The listing builds one solid part. Answer for the finished solid, in the listing's coordinates (mm). Face numbers are marked on the shaded views. A direction names the side the tool comes from. Coordinates: 2 decimals unless noted, no trailing zeros. Order: outer loops, then holes, each group sorted by start corner. A loop starts at its lowest first (then second) coordinate and runs counter-clockwise, first axis right, second up. Notation, with made-up numbers: (62.25, -5.5) -> (97.25, -5.5) arc R6 ccw to (97.25, -1.5) -> close; hole circle Ø4 at (78.5, 6.5). An arc over 180 degrees is marked (long way). Write each question's results on one line, items separated by ' | '. Start each with the question number.
(1) The part is cut by section B-B, the plane x = -15. Give the vertices of the cut face in (y, z).
(2) The part is cut by section D-D, the plane y = 30. Give the vertices of the cut face in (x, z), then the cut area to 3 significant figures.
(3) A tool of negligible diameter and unlimited length cuts with its end or side. For the marked faces 4, 5, 6 and 7, from which of +Z, -Z, +X, -X, +Y, -Y can it reach the whole face along a straight path? Write none if from no direction.
(4) Determine the mould class of the marked faces 1, 2 and 3 for opening direction Z: +Z half, -Z half, draft (parallel to the pull), parting line (faces both ways), or undercut.
(5) Straight lines are drawn through the part: L1, parallel to Z at x = -15, y = 7.5; L2, parallel to Y at x = -14, z = 3.5; L3, parallel to Z at x = -17.5, y = 24.5. For each, find the intervals that lie inside material, in ascending order.
(6) The part is cut by section A-A, the plane z = 0. Give the vertices of the cut face in (x, y).
(7) Given pin 1 (5 mm diameter, centred on x = -15, z = 0, fed in from -Y); pin 2 (8 mm diameter, centred on x = -21, z = -4, fed in from +Y); pin 3 (11 mm diameter, centred on y = 16.5, z = 1, fed in from +X); pin 4 (12 mm diameter, centred on x = -29.5, z = -11.5, fed in from -Y), each flat-ended and moving along its own axis, determine where each tip first touches the part or whether it passes through.
(8) The part is cut by section C-C, the plane z = -9.5. Give the vertices of the cut face in (x, y), then the cut area to 3 significant figures.
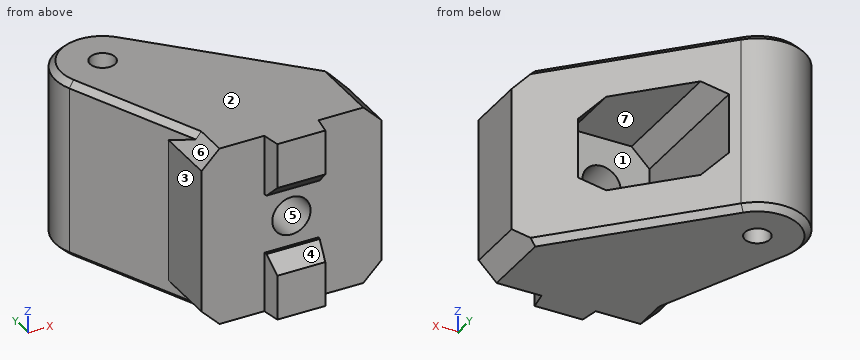
```python
from build123d import *

# Parameters (mm, degrees)
CROQUIS1_R              = 2.1
SALIENTE_EXTRUIR1_DEPTH = 15
CHAFL_N1_SIZE           = 3
CORTAR_EXTRUIR1_START   = -10
CROQUIS3_W              = 16
CROQUIS3_H              = 16
CORTAR_EXTRUIR1_DEPTH   = 28.9
CHAFL_N2_SIZE           = 3
CROQUIS4_R              = 3.2
CORTAR_EXTRUIR2_DEPTH   = 14
CROQUIS5_W              = 10
CROQUIS5_H              = 10
CORTAR_EXTRUIR3_DEPTH   = 4
CHAFL_N3_SIZE           = 2.5
CHAFL_N4_SIZE           = 1


with BuildPart() as part:
    # Croquis1 → Saliente-Extruir1 (new body, symmetric)
    with BuildSketch(Plane.XY):
        with BuildLine():
            Line((-30, 0), (-30, 10))
            Line((-30, 10), (-37.257580847, 26.8795))
            ThreePointArc((-37.257580847, 26.8795), (-34.35566426, 36.590765423), (-24.284119395, 35.453320907))
            Line((-24.284119395, 35.453320907), (0, 10))
            Line((0, 10), (0, 0))
            Line((0, 0), (-10.471019058, 0))
            Line((-10.471019058, 0), (-11, -3))
            Line((-11, -3), (-19, -3))
            Line((-19, -3), (-19.528980942, 0))
            Line((-19.528980942, 0), (-30, 0))
        make_face()
        with Locations((-30, 30)):
            Circle(CROQUIS1_R, mode=Mode.SUBTRACT)
    extrude(amount=SALIENTE_EXTRUIR1_DEPTH, both=True)

    # Chaflán1
    chafl_n1_edges = [part.edges().sort_by_distance(p)[0] for p in [
        (-30, 5, -15),
        (0, 5, -15),
        (-30, 5, 15),
        (0, 5, 15),
    ]]
    chamfer(chafl_n1_edges, length=CHAFL_N1_SIZE)

    # Croquis3 → Cortar-Extruir1 (cut, through all)
    with BuildSketch(Plane.XZ.offset(CORTAR_EXTRUIR1_START)):
        with Locations((-15, 0)):
            Rectangle(CROQUIS3_W, CROQUIS3_H)
    extrude(amount=-CORTAR_EXTRUIR1_DEPTH, mode=Mode.SUBTRACT)

    # Chaflán2
    chafl_n2_edges = [part.edges().sort_by_distance(p)[0] for p in [
        (-23, 22.053687666, -8),
        (-23, 22.053687666, 8),
        (-7, 13.668513637, 8),
        (-7, 13.668513637, -8),
    ]]
    chamfer(chafl_n2_edges, length=CHAFL_N2_SIZE)

    # Croquis4 → Cortar-Extruir2 (cut, through all)
    with BuildSketch(Plane(origin=(0, 10, 0), x_dir=(1, 0, 0), z_dir=(0, 1, 0))):
        with Locations((-15, 0)):
            Circle(CROQUIS4_R)
    extrude(amount=-CORTAR_EXTRUIR2_DEPTH, mode=Mode.SUBTRACT)

    # Croquis5 → Cortar-Extruir3 (cut, through all)
    with BuildSketch(Plane.XZ):
        with Locations((-15, 0)):
            Rectangle(CROQUIS5_W, CROQUIS5_H)
    extrude(amount=CORTAR_EXTRUIR3_DEPTH, mode=Mode.SUBTRACT)

    # Chaflán3
    chafl_n3_edges = [part.edges().sort_by_distance(p)[0] for p in [
        (-15, -3, -5),
        (-15, -3, 5),
    ]]
    chamfer(chafl_n3_edges, length=CHAFL_N3_SIZE)

    # Chaflán4
    chafl_n4_edges = [part.edges().sort_by_distance(p)[0] for p in [
        (-32.128790423, 14.951087519, -15),
        (-34.35566426, 36.590765423, -15),
        (-34.35566426, 36.590765423, 15),
        (-32.128790423, 14.951087519, 15),
        (-13.642059698, 24.298880584, -15),
        (-13.642059698, 24.298880584, 15),
    ]]
    chamfer(chafl_n4_edges, length=CHAFL_N4_SIZE)


solid = part.part
```
Established:
1) outline: (-3, -15) -> (24.27, -15) -> (25.72, -14) -> (25.72, -8) -> (10, -8) -> (10, -3.2) -> (0, -3.2) -> (0, -5) -> (-0.5, -5) -> (-3, -7.5) -> close; (-3, 7.5) -> (-0.5, 5) -> (0, 5) -> (0, 3.2) -> (10, 3.2) -> (10, 8) -> (25.72, 8) -> (25.72, 14) -> (24.27, 15) -> (-3, 15) -> close
2) outline: (-37.9, -14) -> (-36.9, -15) -> (-32.1, -15) -> (-32.1, 15) -> (-36.9, 15) -> (-37.9, 14) -> close; (-27.9, -15) -> (-20.46, -15) -> (-19.08, -14) -> (-19.08, -8) -> (-20, -8) -> (-23, -5) -> (-23, 5) -> (-20, 8) -> (-19.08, 8) -> (-19.08, 14) -> (-20.46, 15) -> (-27.9, 15) -> close | area: 382 mm^2
3) face 4: +X, -X, -Y | face 5: +Y, -Y | face 6: +Z, -X, -Y | face 7: +Y
4) face 1: undercut | face 2: +Z half | face 3: draft
5) L1: z = -15 to -3.2, 3.2 to 15 | L2: y = 0 to 10 | L3: z = -15 to -8, 8 to 15
6) outline: (-37.26, 26.88) -> (-30, 10) -> (-30, 0) -> (-18.2, 0) -> (-18.2, 10) -> (-23, 10) -> (-23, 34.11) -> (-24.28, 35.45) arc R7.9 ccw to start; (-11.8, 0) -> (0, 0) -> (0, 10) -> (-7, 17.34) -> (-7, 10) -> (-11.8, 10) -> close; hole circle Ø4.2 at (-30, 30)
7) pin 1: passes through | pin 2: stops at y = 36.12 | pin 3: stops at x = -0.95 | pin 4: stops at y = 0
8) outline: (-37.26, 26.88) -> (-30, 10) -> (-30, 0) -> (-19.53, 0) -> (-19, -3) -> (-11, -3) -> (-10.47, 0) -> (0, 0) -> (0, 10) -> (-24.28, 35.45) arc R7.9 ccw to start; hole circle Ø4.2 at (-30, 30) | area: 910 mm^2
